from build123d import *

# Parameters (mm, degrees)
F0_W     = 250
F0_H     = 15
F1_DEPTH = 13
F1_TAPER = -3
F3_D     = 5.5
F4_D     = 10
F4_DEPTH = 8
F4_TIP   = 3.0043030951


with BuildPart() as f1:
    # F0 (on Top) → F1 (new body)
    with BuildSketch(Plane.XY):
        with Locations((-13.7262433767, 28.3889581655)):
            Rectangle(F0_W, F0_H)
    extrude(amount=F1_DEPTH, taper=F1_TAPER)

    # F3 (through all)
    with Locations(Plane(origin=(0, 0, 0), x_dir=(1, 0, 0), z_dir=(0, 0, -1))):
        with Locations((-131.4075445074, -29.0702592962), (-37.4075445074, -29.0702592962), (9.9550577539, -29.0702592962), (103.9550577539, -29.0702592962)):
            Hole(F3_D / 2)

    # F4
    with Locations(Plane(origin=(0, 0, 0), x_dir=(1, 0, 0), z_dir=(0, 0, -1))):
        with Locations((-37.4075445074, -29.0702592962), (9.9550577539, -29.0702592962), (103.9550577539, -29.0702592962), (-131.4075445074, -29.0702592962)):
            Hole(F4_D / 2, depth=F4_DEPTH)
            with Locations((0, 0, -(F4_DEPTH + F4_TIP / 2))):  # 118° drill point
                Cone(0, F4_D / 2, F4_TIP, mode=Mode.SUBTRACT)


solid = f1.part
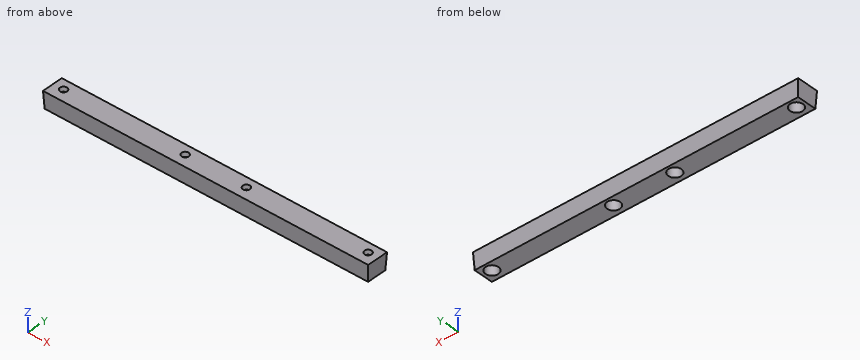
Geometry: final body of the model. Coordinates: model frame, mm. Give positions to 0.01 mm unless a question says otherwise; leave off trailing zeros. Return JSON: item names as keys, results as strings. Group by question number.
1) Line query: line 1 (X direction, y = 32, z = 3.75); line 2 (X direction, y = 29.5, z = 1.5); line 3 (Y direction, x = -124, z = 0.5). Output: solid intervals per line, ascending.
2) Section A-A on z = 2.5. State how many separate pieces and enclosed holes the cut face has, plus the area to 3 significant figures.
3) First-contact query: P1, Ø6, axis at y = 26.5, z = 1.5, coming from the +X side; P2, Ø5, axis at x = -102, y = 32.5, coming from the -Z side; P3, Ø1, axis at x = -52, z = 8, coming from the +Y side; P4, Ø6.5, axis at x = 9.96, y = 29.07, coming from the -Z side. Flat tips, straight axial feed; report the tip coordinate or a pass-through.
Filled in:
{
 "1": {"line 1": "x = -138.92 to -135.46, -127.36 to -41.46, -33.36 to 5.9, 14.01 to 99.9, 108.01 to 111.47", "line 2": "x = -138.8 to -136.39, -126.43 to -42.39, -32.43 to 4.97, 14.94 to 98.97, 108.94 to 111.35", "line 3": "y = 20.86 to 35.92"},
 "2": {"separate pieces": "1", "enclosed holes": "4", "area": "3,510 mm^2"},
 "3": {"P1": "stops at x = 111.51", "P2": "stops at z = 0", "P3": "stops at y = 36.33", "P4": "stops at z = 9.05"}
}
